```python
from build123d import *

# Parameters (mm, degrees)
SKETCH_1_W                      = 136
SKETCH_1_H                      = 104
EXTRUDE_1_DEPTH                 = 42
SKETCH_2_W                      = 116
SKETCH_2_H                      = 84
CUT_EXTRUDE_1_DEPTH             = 36
CUT_EXTRUDE_2_REACH             = 94.865
SKETCH_3_R                      = 5
SKETCH_5_R                      = 5
CUT_EXTRUDE_4_DEPTH             = 104
SKETCH_6_W                      = 10
SKETCH_6_H                      = 20
EXTRUDE_2_DEPTH                 = 258
SKETCH_8_W                      = 20
SKETCH_8_H                      = 30
EXTRUDE_4_DEPTH                 = 10
SKETCH_9_W                      = 10
SKETCH_9_H                      = 20
EXTRUDE_5_DEPTH                 = 129
SKETCH_10_W                     = 20
SKETCH_10_H                     = 30
EXTRUDE_6_DEPTH                 = 10
SKETCH_12_W                     = 10
SKETCH_12_H                     = 20
EXTRUDE_8_DEPTH                 = 129
SKETCH_13_W                     = 20
SKETCH_13_H                     = 129
CUT_EXTRUDE_5_DEPTH             = 10
SKETCH_14_W                     = 20
SKETCH_14_H                     = 129
CUT_EXTRUDE_6_DEPTH             = 10
SKETCH_15_R                     = 10
EXTRUDE_9_DEPTH                 = 156
CUT_EXTRUDE_7_REACH             = 344.491
SKETCH_16_R                     = 2.2
CUT_EXTRUDE_7_DIRECTION_2_DEPTH = 136


with BuildPart() as part:
    # 草图1 → 凸台-拉伸1 (new body)
    with BuildSketch(Plane(origin=(0, 0, 0), x_dir=(1, 0, 0), z_dir=(0, 1, 0))):
        Rectangle(SKETCH_1_W, SKETCH_1_H)
    extrude(amount=EXTRUDE_1_DEPTH)

    # 草图2 → 切除-拉伸1 (cut)
    with BuildSketch(Plane(origin=(0, 42, 0), x_dir=(1, 0, 0), z_dir=(0, 1, 0))):
        Rectangle(SKETCH_2_W, SKETCH_2_H)
    extrude(amount=-CUT_EXTRUDE_1_DEPTH, mode=Mode.SUBTRACT)

    # 草图3 → 切除-拉伸2 (cut, up to next)
    with BuildSketch(Plane(origin=(0, 6, 0), x_dir=(1, 0, 0), z_dir=(0, 1, 0)), mode=Mode.PRIVATE) as cut_extrude_2_sk1:
        with Locations(Location((-34, 0, 0), (0, 0, 270))):
            Circle(SKETCH_3_R)
    cut_extrude_2_tool1 = extrude(cut_extrude_2_sk1.sketch, amount=-CUT_EXTRUDE_2_REACH, mode=Mode.PRIVATE) & part.part
    # 草图3 → 切除-拉伸2 (cut, up to next)
    with BuildSketch(Plane(origin=(0, 6, 0), x_dir=(1, 0, 0), z_dir=(0, 1, 0)), mode=Mode.PRIVATE) as cut_extrude_2_sk2:
        with Locations(Location((34, 0, 0), (0, 0, 270))):
            Circle(SKETCH_3_R)
    cut_extrude_2_tool2 = extrude(cut_extrude_2_sk2.sketch, amount=-CUT_EXTRUDE_2_REACH, mode=Mode.PRIVATE) & part.part
    add(cut_extrude_2_tool1.solids().sort_by_distance((-34, 6, 0))[0], mode=Mode.SUBTRACT)
    add(cut_extrude_2_tool2.solids().sort_by_distance((34, 6, 0))[0], mode=Mode.SUBTRACT)

    # 草图5 → 切除-拉伸4 (cut)
    with BuildSketch(Plane.XY.offset(52)):
        with Locations((0, 21)):
            Circle(SKETCH_5_R)
    extrude(amount=-CUT_EXTRUDE_4_DEPTH, mode=Mode.SUBTRACT)

    # 草图6 → 凸台-拉伸2 (add)
    with BuildSketch(Plane(origin=(0, 42, 0), x_dir=(1, 0, 0), z_dir=(0, 1, 0))):
        with Locations((-63, 0)):
            Rectangle(SKETCH_6_W, SKETCH_6_H)
        with Locations((63, 0)):
            Rectangle(SKETCH_6_W, SKETCH_6_H)
    extrude(amount=EXTRUDE_2_DEPTH)

    # 草图8 → 凸台-拉伸4 (add)
    with BuildSketch(Plane.ZY.offset(68)):
        with Locations((0, 156)):
            Rectangle(SKETCH_8_W, SKETCH_8_H)
    extrude(amount=EXTRUDE_4_DEPTH)

    # 草图9 → 凸台-拉伸5 (add)
    with BuildSketch(Plane(origin=(0, 171, 0), x_dir=(1, 0, 0), z_dir=(0, 1, 0))):
        with Locations((-73, 0)):
            Rectangle(SKETCH_9_W, SKETCH_9_H)
    extrude(amount=EXTRUDE_5_DEPTH)

    # 草图10 → 凸台-拉伸6 (add)
    with BuildSketch(Plane(origin=(68, 0, 0), x_dir=(0, 0, -1), z_dir=(1, 0, 0))):
        with Locations((0, 156)):
            Rectangle(SKETCH_10_W, SKETCH_10_H)
    extrude(amount=EXTRUDE_6_DEPTH)

    # 草图12 → 凸台-拉伸8 (add)
    with BuildSketch(Plane(origin=(0, 171, 0), x_dir=(1, 0, 0), z_dir=(0, 1, 0))):
        with Locations((73, 0)):
            Rectangle(SKETCH_12_W, SKETCH_12_H)
    extrude(amount=EXTRUDE_8_DEPTH)

    # 草图13 → 切除-拉伸5 (cut)
    with BuildSketch(Plane(origin=(-58, 0, 0), x_dir=(0, 0, -1), z_dir=(1, 0, 0))):
        with Locations((0, 235.5)):
            Rectangle(SKETCH_13_W, SKETCH_13_H)
    extrude(amount=-CUT_EXTRUDE_5_DEPTH, mode=Mode.SUBTRACT)

    # 草图14 → 切除-拉伸6 (cut)
    with BuildSketch(Plane.ZY.offset(-58)):
        with Locations((0, 235.5)):
            Rectangle(SKETCH_14_W, SKETCH_14_H)
    extrude(amount=-CUT_EXTRUDE_6_DEPTH, mode=Mode.SUBTRACT)

    # 草图15 → 凸台-拉伸9 (add)
    with BuildSketch(Plane.ZY.offset(78)):
        with Locations((0, 300)):
            Circle(SKETCH_15_R)
    extrude(amount=-EXTRUDE_9_DEPTH)

    # 草图16 → 切除-拉伸7 (cut, up to next)
    with BuildSketch(Plane(origin=(-58, 0, 0), x_dir=(0, 0, -1), z_dir=(1, 0, 0)), mode=Mode.PRIVATE) as cut_extrude_7_sk1:
        with Locations((0, 163)):
            Circle(SKETCH_16_R)
    cut_extrude_7_tool1 = extrude(cut_extrude_7_sk1.sketch, amount=-CUT_EXTRUDE_7_REACH, mode=Mode.PRIVATE) & part.part
    # 草图16 → 切除-拉伸7 (cut, up to next)
    with BuildSketch(Plane(origin=(-58, 0, 0), x_dir=(0, 0, -1), z_dir=(1, 0, 0)), mode=Mode.PRIVATE) as cut_extrude_7_sk2:
        with Locations((0, 149)):
            Circle(SKETCH_16_R)
    cut_extrude_7_tool2 = extrude(cut_extrude_7_sk2.sketch, amount=-CUT_EXTRUDE_7_REACH, mode=Mode.PRIVATE) & part.part
    add(cut_extrude_7_tool1.solids().sort_by_distance((-58, 163, 0))[0], mode=Mode.SUBTRACT)
    add(cut_extrude_7_tool2.solids().sort_by_distance((-58, 149, 0))[0], mode=Mode.SUBTRACT)

    # 草图16 → 切除-拉伸7 direction 2 (cut)
    with BuildSketch(Plane(origin=(-58, 0, 0), x_dir=(0, 0, -1), z_dir=(1, 0, 0))):
        with Locations((0, 163)):
            Circle(SKETCH_16_R)
        with Locations((0, 149)):
            Circle(SKETCH_16_R)
    extrude(amount=CUT_EXTRUDE_7_DIRECTION_2_DEPTH, mode=Mode.SUBTRACT)


solid = part.part
```
Input: part model. Units: mm. Frame: model coordinates. A direction names the side the tool comes from. Give positions to 0.01 mm unless a question says otherwise; leave off trailing zeros. Write each loop counter-clockwise with the first axis right and the second up, starting at its lowest first coordinate (ties: lowest second). Pieces come first, ordered by that corner, then holes. Notation, with made-up numbers: (0, 63) - (9, 63) arc R5 ccw to (9, 72) - close; hole circle Ø2 at (27, -15.5). An arc over 180 degrees is marked (long way). Write item = value, one per line. Start each with the question number.
1) Cut plane D-D (x = 34). Return loops of the section in (y, z).
2) Draft query along X for faces 6 (the face through (-38.88, 3.04, -1.08)), 7 (the face through (68, 38, 1)), 8 (the face through (68, 169, -10)), 9 (the face through (38.957, 3.042, -0.651)). Return one class per face: pulls with the +X half, pulls with the -X half, needs draft (parallel to the pull), parting line crosses it, or undercut.
3) Cut plane A-A (y = 187.5). Return loops of the section in (x, z), and give its area (3 significant figures).
4) Cut plane B-B (x = 12). Return loops of the section in (y, z), and give its area (3 significant figures).
5) Material intervals for L1, parallel to Y at x = -67.5, z = 0; L2, parallel to X at y = 2.2, z = 0; L3, parallel to X at y = 121.5, z = -2, sorted ascending. Write a range as [from, to].
6) Reachability of faces 1 (the face through (-1, 28, 42)), 2 (the face through (-68, 169, 10)), 3 (the face through (73, 141, 0)), 4 (the face through (-68, 38, 1)), 5 (the face through (-58, 71, 1)) from +Z, -Z, +X, -X, +Y, -Y: full face, straight path, thin tool, end or side. Return the list, or none.
7) Cut plane C-C (z = 45). Return loops of the section in (x, y).
8) Pin query (flat end, axial travel): pin 1 (4 mm diameter, centred on y = 149, z = 0, fed in from +X); pin 2 (11 mm diameter, centred on x = -74.5, z = -3, fed in from -Y); pin 3 (1.5 mm diameter, centred on x = -28.5, z = -39, fed in from +Y); pin 4 (10 mm diameter, centred on x = -63.5, y = 154, fed in from +Z). Return the tip coordinate at first contact, or that it passes through.
Answers follow:
q1.outline = (0, -52) - (42, -52) - (42, -42) - (6, -42) - (6, -5) - (0, -5) - close; (0, 5) - (6, 5) - (6, 42) - (42, 42) - (42, 52) - (0, 52) - close; circle Ø20 at (300, 0)
q2.face_6 = undercut
q2.face_7 = pulls with the +X half
q2.face_8 = needs draft
q2.face_9 = undercut
q3.outline = (-78, -10) - (-68, -10) - (-68, 10) - (-78, 10) - close; (68, -10) - (78, -10) - (78, 10) - (68, 10) - close
q3.area = 400 mm^2
q4.outline = (0, -52) - (42, -52) - (42, -42) - (6, -42) - (6, 42) - (42, 42) - (42, 52) - (0, 52) - close; circle Ø20 at (300, 0)
q4.area = 1,660 mm^2
q5.L1 = [0, 146.8], [151.2, 160.8], [165.2, 171], [290, 310]
q5.L2 = [-68, -39], [-29, 29], [39, 68]
q5.L3 = [-68, -58], [58, 68]
q6.face_1 = +Y
q6.face_2 = +Z, +X, -X, +Y
q6.face_3 = +Z, -Z, +X, -Y
q6.face_4 = +Z, -Z, -X, -Y
q6.face_5 = none
q7.outline = (-68, 0) - (68, 0) - (68, 42) - (-68, 42) - close; hole circle Ø10 at (0, 21)
q8.pin_1 = through
q8.pin_2 = 141
q8.pin_3 = 6
q8.pin_4 = 10
